Can you work these out from the model? Positions are in its coordinate system, mm. A direction names the side the tool comes from. Coordinates: 2 decimals unless noted, no trailing zeros. Order: outer loops, then holes, each group sorted by start corner. A loop starts at its lowest first (then second) coordinate and runs counter-clockwise, first axis right, second up. Notation, with made-up numbers: (-20.75, -34.5) -> (7.25, -34.5) arc R16 cw to (7.25, -24.5) -> close; hole circle Ø1 at (16, 35.5). An arc over 180 degrees is marked (long way). Write item = value, one per line.
```python
from build123d import *

# Parameters (mm, degrees)
F2_W     = 0.79375
F2_H     = 12.7
F3_DEPTH = 12.7


with BuildPart() as f1:
    # F0 (on Front) → F1 (revolve)
    with BuildSketch(Plane.XZ):
        Polygon((3.571875, 0), (5.159375, 0), (5.159375, 28.575), (1.5875, 41.275), (0.79375, 41.275), (0.79375, 2.778125), align=None)
    revolve(axis=Axis((0, 0, 23.459722), (0, 0, -1)))

    # F2 (on Front) → F3 (cut, symmetric)
    with BuildSketch(Plane.XZ):
        with Locations((-4.7625, 19.05)):
            Rectangle(F2_W, F2_H)
        with Locations((4.7625, 19.05)):
            Rectangle(F2_W, F2_H)
    extrude(amount=F3_DEPTH, both=True, mode=Mode.SUBTRACT)


solid = f1.part
```
Item 1: I'm going to push flat-ended pins straight in: P1, Ø1, axis at x = 2.5, z = 29.5, coming from the -Y side; P2, Ø2, axis at x = 1.5, z = 37, coming from the +Y side; P3, Ø1.6, axis at y = -1, z = 21.5, coming from the -X side. Where does each tip first touch, or does it pass through?
A:
P1 = -4.52
P2 = 2.88
P3 = -4.37
Item 2: If we mould it in two halves opening along X, with no side actions, what happens to faces 3 (the cylindrical face through (-0.172, 0.775, 21.757)), 4 (the flat face through (4.366, 0, 19)), 5 (the conical face through (0.923, -0.291, 2.604)), 6 (the conical face through (1.36, 2.62, 36.43))? For each: pulls with the +X half, pulls with the -X half, needs draft (parallel to the pull), parting line crosses it, or undercut.
A:
face_3 = undercut
face_4 = pulls with the +X half
face_5 = undercut
face_6 = parting line crosses it
Item 3: I want a section at D-D, the plane z = 5. Please give me the cut outline in (x, y).
A:
outline = circle Ø10.32 at (0, 0); hole circle Ø1.59 at (0, 0)
Item 4: I want a section at C-C, the plane z = 19. Please give me the cut outline in (x, y).
A:
outline = (-4.37, -2.75) arc R5.16 ccw to (4.37, -2.75) -> (4.37, 2.75) arc R5.16 ccw to (-4.37, 2.75) -> close; hole circle Ø1.59 at (0, 0)
Item 5: I want a section at B-B, the plane x = 0. Please give me the cut outline in (y, z) (1 decimal).
A:
outline = (-5.2, 0) -> (-3.6, 0) -> (-0.8, 2.8) -> (-0.8, 41.3) -> (-1.6, 41.3) -> (-5.2, 28.6) -> close; (0.8, 2.8) -> (3.6, 0) -> (5.2, 0) -> (5.2, 28.6) -> (1.6, 41.3) -> (0.8, 41.3) -> close
Item 6: I want a section at A-A, the plane y = 0. Please give me the cut outline in (x, z) (1 decimal), plus the area to 3 significant figures.
A:
outline = (-5.2, 0) -> (-3.6, 0) -> (-0.8, 2.8) -> (-0.8, 41.3) -> (-1.6, 41.3) -> (-5.2, 28.6) -> (-5.2, 25.4) -> (-4.4, 25.4) -> (-4.4, 12.7) -> (-5.2, 12.7) -> close; (0.8, 2.8) -> (3.6, 0) -> (5.2, 0) -> (5.2, 12.7) -> (4.4, 12.7) -> (4.4, 25.4) -> (5.2, 25.4) -> (5.2, 28.6) -> (1.6, 41.3) -> (0.8, 41.3) -> close
area = 287 mm2
Item 7: If I drill on probe 1 along Y at (x, z) = (0, 12); probe 2 along X at (y, z) = (0, 21); probe 3 along X at (y, z) = (-1.5, 20), over which ranges is the centre line in solid material (lowest first)?
A:
probe_1 = -5.16 to -0.79, 0.79 to 5.16
probe_2 = -4.37 to -0.79, 0.79 to 4.37
probe_3 = -4.37 to 4.37
Item 8: For faces 1 (the flat face through (-4.366, 0, 19)), 2 (the cylindrical face through (-4.094, 3.139, 14.488)), which set-ups out of +Z, -Z, +X, -X, +Y, -Y let a thin tool reach every point of the face, with its end or its side?
A:
face_1 = -X, +Y, -Y
face_2 = +Z, -Z
